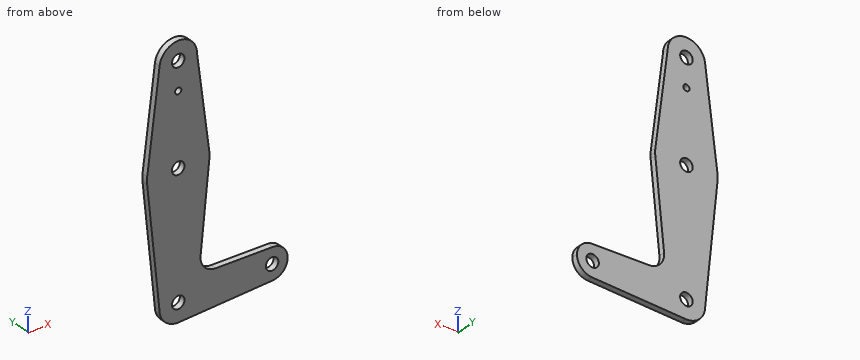
```python
from build123d import *

# Parameters (mm, degrees)
F0_R     = 3.175
F0_R_2   = 1.5875
F1_DEPTH = 3.048


with BuildPart() as f1:
    # F0 (on Front) → F1 (new body)
    with BuildSketch(Plane.XZ):
        with BuildLine():
            ThreePointArc((0.632547, -9.503973), (6.955237, -6.507711), (9.525, 0))
            ThreePointArc((9.525, 0), (0, 9.525), (-9.525, 0))
            ThreePointArc((-9.525, 0), (-6.735192, -6.735192), (0, -9.525))
            Line((0, -9.525), (0.632547, -9.503973))
        make_face()
        Circle(F0_R, mode=Mode.SUBTRACT)
        with BuildLine():
            ThreePointArc((-9.525, 0), (0, 9.525), (9.525, 0))
            ThreePointArc((9.525, 0), (6.955237, -6.507711), (0.632547, -9.503973))
            Line((0.632547, -9.503973), (47.888707, -7.933118))
            ThreePointArc((47.888707, -7.933118), (39.6875, 0.000438), (47.889583, 7.933089))
            Line((47.889583, 7.933089), (18.990985, 8.896911))
            ThreePointArc((18.990985, 8.896911), (13.271886, 11.608559), (11.345642, 17.637713))
            Line((11.345642, 17.637713), (15.795426, 61.9125))
            ThreePointArc((15.795426, 61.9125), (0.006091, 47.625001), (-15.794203, 61.90038))
            Line((-15.794203, 61.90038), (-9.525, 0))
        make_face()
        with BuildLine():
            ThreePointArc((0, -9.525), (0.316448, -9.519742), (0.632547, -9.503973))
            Line((0.632547, -9.503973), (0, -9.525))
        make_face()
        with BuildLine():
            ThreePointArc((-15.750488, 65.484375), (-15.873819, 63.693615), (-15.794203, 61.90038))
            ThreePointArc((-15.794203, 61.90038), (0.006091, 47.625001), (15.795426, 61.9125))
            ThreePointArc((15.795426, 61.9125), (15.855094, 62.705253), (15.875, 63.5))
            ThreePointArc((15.875, 63.5), (15.843082, 64.506168), (15.747457, 65.508289))
            ThreePointArc((15.747457, 65.508289), (-0.012053, 79.374995), (-15.750488, 65.484375))
        make_face()
        with Locations((0, 63.5)):
            Circle(F0_R, mode=Mode.SUBTRACT)
        with BuildLine():
            ThreePointArc((47.889583, 7.933089), (39.6875, 0.000438), (47.888707, -7.933118))
            ThreePointArc((47.888707, -7.933118), (53.330133, -5.518638), (55.5625, 0))
            ThreePointArc((55.5625, 0), (53.330438, 5.518323), (47.889583, 7.933089))
        make_face()
        with Locations((47.625, 0)):
            Circle(F0_R, mode=Mode.SUBTRACT)
        with BuildLine():
            Line((-9.450293, 115.490625), (-15.750488, 65.484375))
            ThreePointArc((-15.750488, 65.484375), (-0.012053, 79.374995), (15.747457, 65.508289))
            Line((15.747457, 65.508289), (9.525, 114.3))
            ThreePointArc((9.525, 114.3), (-0.596483, 104.793695), (-9.450293, 115.490625))
        make_face()
        with Locations((0, 100.0252)):
            Circle(F0_R_2, mode=Mode.SUBTRACT)
        with BuildLine():
            ThreePointArc((9.525, 114.3), (0.596483, 123.806305), (-9.450293, 115.490625))
            ThreePointArc((-9.450293, 115.490625), (-0.596483, 104.793695), (9.525, 114.3))
        make_face()
        with Locations((0, 114.3)):
            Circle(F0_R, mode=Mode.SUBTRACT)
    extrude(amount=F1_DEPTH)


solid = f1.part
```
Geometry: final body of the model. Coordinates: model frame, mm. Give positions to 0.01 mm unless a question says otherwise; leave off trailing zeros. Write each loop counter-clockwise with the first axis right and the second up, starting at its lowest first coordinate (ties: lowest second). Pieces come first, ordered by that corner, then holes.
1. Section query D-D, the plane x = -5. Return loops of the section in (y, z).
2. Pin query (flat end, axial travel): P1, Ø5, axis at x = 0, z = 63.5, coming from the -Y side; P2, Ø1, axis at y = -2, z = 12.5, coming from the -X side; P3, Ø1, axis at y = -2, z = 29.5, coming from the +X side. Return the tip coordinate at first contact, or that it passes through.
3. Line query: probe 1 along Z at (x, y) = (48, -1.45); probe 2 along Z at (x, y) = (2, -0.35); probe 3 along X at (y, z) = (-0.25, 100). Output: solid intervals per line, ascending.
4. Section query A-A, the plane x = 14. Return loops of the section in (y, z), then the cut area to 3 significant figures.
5. Section query B-B, the plane y = -0.5. Count the separate pieces of the cut face and the enclosed holes in it, then the cut area to 3 significant figures.
6. Section query C-C, the plane z = 40. Return loops of the section in (x, y), then the cut area to 3 significant figures.
Computed:
1. outline: (-3.05, -8.11) - (0, -8.11) - (0, 122.41) - (-3.05, 122.41) - close
2. P1: passes through
2. P2: stops at x = -10.84
2. P3: stops at x = 12.59
3. probe 1: z = -7.93 to -3.15, 3.15 to 7.93
3. probe 2: z = -9.46 to -2.47, 2.47 to 61.03, 65.97 to 111.83, 116.77 to 123.61
3. probe 3: x = -11.4 to -1.59, 1.59 to 11.35
4. outline: (-3.05, -9.06) - (0, -9.06) - (0, 10.88) - (-3.05, 10.88) - close; (-3.05, 44.05) - (0, 44.05) - (0, 79.21) - (-3.05, 79.21) - close
4. area: 168 mm2
5. separate pieces: 1
5. enclosed holes: 5
5. area: 3,850 mm2
6. outline: (-13.58, -3.05) - (13.59, -3.05) - (13.59, 0) - (-13.58, 0) - close
6. area: 82.8 mm2
